Input: part model. Units: mm. Frame: model coordinates. Round coordinates to 2 decimals unless told otherwise and drop trailing zeros. Loops run counter-clockwise (first coordinate to the right, second up) from the corner with the lowest first, then second, coordinate; pieces in that order, holes last. Notation, with made-up numbers: M 2.5,75.5 L 28.5,75.5 A17 ccw 28.5,104.5 Z; hole C 58.25,-28.5 d5. An arc over 180 degrees is marked long. Use one line per item in the form item = value. Start each with the question number.
Q1. Section query B-B, the plane z = 25.4. Output: boundary loops of the cut face in (x, y), and give its area (3 significant figures).
Q2. Section query A-A, the plane x = 0. Output: boundary loops of the cut face in (y, z), and give its area (3 significant figures).
Q3. Section query C-C, the plane y = -0.75. Output: boundary loops of the cut face in (x, z).
Q4. Mould query, pull axis Z, two halves, no side actions, for faces 1 (the flat face through (0, 0, 38.1)), 2 (the cylindrical face through (2.33, -0.02, -0.31)), 3 (the flat face through (3, -1.588, -1)), 4 (the cylindrical face through (0.71, -0.02, 27.64)). Classes: pulls with the +Z half, pulls with the -Z half, needs draft (parallel to the pull), parting line crosses it, or undercut.
Q5. First-contact query: P1, Ø3, axis at x = 0, z = 25.4, coming from the +Y side. Flat tip, straight axial feed; report the tip coordinate or a pass-through.
Q6. Ray query, line 1 along Z through (x, y) = (0, 0.2); line 2 along X through (y, z) = (0.8, 25.4); line 3 along X through (y, z) = (0.3, -2). Return the intervals inside material, ascending.
```python
from build123d import *

# Parameters (mm, degrees)
SKETCH1_W               = 25.4
SKETCH1_H               = 76.2
BOSS_EXTRUDE1_DEPTH     = 1.5875
CUT_EXTRUDE1_DEPTH      = 41.286233691
CUT_EXTRUDE1_DEPTH_BACK = 41.286233691
SKETCH2_R               = 2.3495


with BuildPart() as part:
    # Sketch1 → Boss-Extrude1 (new, symmetric)
    with BuildSketch(Plane(origin=(0, 0, 0), x_dir=(1, 0, 0), z_dir=(0, 1, 0))):
        Rectangle(SKETCH1_W, SKETCH1_H)
    extrude(amount=BOSS_EXTRUDE1_DEPTH, both=True)

    # Sketch2 → Cut-Extrude1 (cut, two sides: drawn at the far end of the back side and taken through both)
    with BuildSketch(Plane(origin=(0, 1.5875, 0), x_dir=(1, 0, 0), z_dir=(0, 1, 0)).offset(-CUT_EXTRUDE1_DEPTH_BACK)):
        with Locations(Location((0, -25.4, 0), (0, 0, 270))):
            Circle(SKETCH2_R)
        with Locations(Location((0, 0, 0), (0, 0, 270))):
            Circle(SKETCH2_R)
        with Locations(Location((0, 25.4, 0), (0, 0, 270))):
            Circle(SKETCH2_R)
    extrude(amount=CUT_EXTRUDE1_DEPTH + CUT_EXTRUDE1_DEPTH_BACK, mode=Mode.SUBTRACT)


solid = part.part
```
Results found:
q1.outline = M -12.7,-1.59 L -2.35,-1.59 L -2.35,1.59 L -12.7,1.59 Z; M 2.35,-1.59 L 12.7,-1.59 L 12.7,1.59 L 2.35,1.59 Z
q1.area = 65.7 mm²
q2.outline = M -1.59,-38.1 L 1.59,-38.1 L 1.59,-27.75 L -1.59,-27.75 Z; M -1.59,-23.05 L 1.59,-23.05 L 1.59,-2.35 L -1.59,-2.35 Z; M -1.59,2.35 L 1.59,2.35 L 1.59,23.05 L -1.59,23.05 Z; M -1.59,27.75 L 1.59,27.75 L 1.59,38.1 L -1.59,38.1 Z
q2.area = 197 mm²
q3.outline = M -12.7,-38.1 L 12.7,-38.1 L 12.7,38.1 L -12.7,38.1 Z; hole C 0,-25.4 d4.7; hole C 0,0 d4.7; hole C 0,25.4 d4.7
q4.face_1 = pulls with the +Z half
q4.face_2 = undercut
q4.face_3 = needs draft
q4.face_4 = undercut
q5.P1 = through
q6.line_1 = -38.1 to -27.75, -23.05 to -2.35, 2.35 to 23.05, 27.75 to 38.1
q6.line_2 = -12.7 to -2.35, 2.35 to 12.7
q6.line_3 = -12.7 to -1.23, 1.23 to 12.7
